```python
from build123d import *

# Parameters (mm, degrees)
BOSS_EXTRUDE1_DEPTH = 10
SKETCH2_R           = 3
CUT_EXTRUDE1_DEPTH  = 10
SKETCH4_R           = 11
CUT_EXTRUDE3_DEPTH  = 8
SKETCH5_R           = 3
SKETCH5_R_2         = 1.5
CUT_EXTRUDE4_DEPTH  = 8
SKETCH7_W           = 21.5
SKETCH7_H           = 2
BOSS_EXTRUDE2_DEPTH = 12
FILLET1_R           = 5
SKETCH8_R           = 3
CUT_EXTRUDE5_DEPTH  = 20
FILLET2_R           = 5


with BuildPart() as part:
    # Sketch1 → Boss-Extrude1 (new body)
    with BuildSketch(Plane(origin=(0, 0, 0), x_dir=(1, 0, 0), z_dir=(0, 1, 0))):
        Polygon((5.5, 11), (5.5, 26), (-26, 26), (-26, -16), (5.5, -16), (5.5, -11), (17.5, -11), (17.5, 11), align=None)
    extrude(amount=BOSS_EXTRUDE1_DEPTH)

    # Sketch2 → Cut-Extrude1 (cut)
    with BuildSketch(Plane(origin=(17.5, 0, 0), x_dir=(0, 0, -1), z_dir=(1, 0, 0))):
        with Locations((-6, 5)):
            Circle(SKETCH2_R)
        with Locations((6, 5)):
            Circle(SKETCH2_R)
    extrude(amount=-CUT_EXTRUDE1_DEPTH, mode=Mode.SUBTRACT)

    # Sketch4 → Cut-Extrude3 (cut)
    with BuildSketch(Plane.XZ):
        with Locations(Location((-11.695464036, 0, 0), (0, 0, 270))):
            Circle(SKETCH4_R)
    extrude(amount=-CUT_EXTRUDE3_DEPTH, mode=Mode.SUBTRACT)

    # Sketch5 → Cut-Extrude4 (cut)
    with BuildSketch(Plane(origin=(0, 8, 0), x_dir=(-1, 0, 0), z_dir=(0, -1, 0))):
        with Locations(Location((11.695464036, 0, 0), (0, 0, 90))):
            Circle(SKETCH5_R)
        with Locations(Location((11.695464036, -6.25, 0), (0, 0, 90))):
            Circle(SKETCH5_R_2)
        with Locations(Location((11.695464036, 6.25, 0), (0, 0, 90))):
            Circle(SKETCH5_R_2)
    extrude(amount=-CUT_EXTRUDE4_DEPTH, mode=Mode.SUBTRACT)

    # Sketch7 → Boss-Extrude2 (add)
    with BuildSketch(Plane(origin=(0, 0, 0), x_dir=(-1, 0, 0), z_dir=(0, -1, 0))):
        with Locations((10.25, 25)):
            Rectangle(SKETCH7_W, SKETCH7_H)
    extrude(amount=BOSS_EXTRUDE2_DEPTH)

    # Fillet1
    fillet1_edges = [part.edges().sort_by_distance(p)[0] for p in [
        (-26, 5, -26),
        (5.5, 5, -26),
        (5.5, 5, 16),
        (-26, 5, 16),
    ]]
    fillet(fillet1_edges, radius=FILLET1_R - 0.0001)  # a hair under: the kernel refuses the full size

    # Sketch8 → Cut-Extrude5 (cut)
    with BuildSketch(Plane.XY.offset(-24)):
        with Locations((-16, -5)):
            Circle(SKETCH8_R)
        with Locations((-4.5, -5)):
            Circle(SKETCH8_R)
    extrude(amount=-CUT_EXTRUDE5_DEPTH, mode=Mode.SUBTRACT)

    # Fillet2
    fillet2_edges = [part.edges().sort_by_distance(p)[0] for p in [
        (0.5, -12, -25),
        (-21, -12, -25),
    ]]
    fillet(fillet2_edges, radius=FILLET2_R)


solid = part.part
```
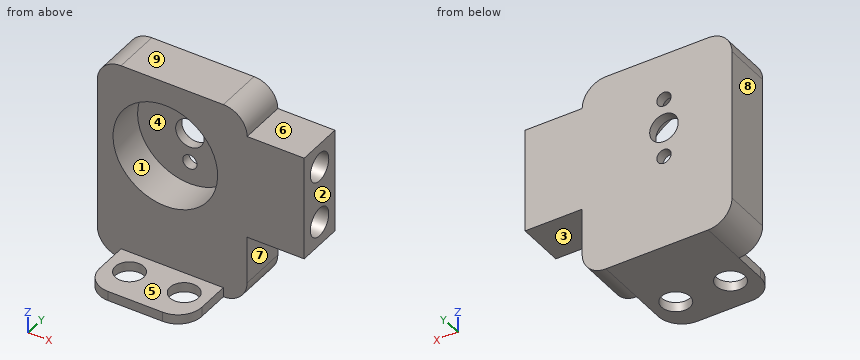
Design review of the part built by this model. Coordinates are the model's own, in mm. Face numbers are marked on the shaded views. A direction names the side the tool comes from. Give positions to 0.01 mm unless a question says otherwise; leave off trailing zeros. Order: outer loops, then holes, each group sorted by start corner. A loop starts at its lowest first (then second) coordinate and runs counter-clockwise, first axis right, second up. Notation, with made-up numbers: (-13, 52) - (24, 52) arc R17 cw to (24, 74) - close; hole circle Ø1 at (43, -15). An arc over 180 degrees is marked (long way). Use a Markdown table: item, result. Add a question column.
(1) Machinability: for the marked faces 5, 6, 7, 8 and 9, which of the approach directions +Z, -Z, +X, -X, +Y, -Y give a long, thin tool a straight path to every point of the face, cutting with its end or side? Answer none if there is none.
(2) Clearance check with flat-ended pins moving along their axes: P1, Ø1, axis at x = -6.5, y = -2, coming from the +Z side; P2, Ø13, axis at x = -11.7, z = 0, coming from the -Y side; P3, Ø12, axis at x = 1, z = 10.5, coming from the -Y side. State where each tip first meets the part, or that it passes through.
(3) Add section D-D on z = 6. Give the boundary of the cut face in (x, y) (3 decimals), then the cut area to 3 significant figures.
(4) Add section A-A on y = -5. Give the boundary of the cut face in (x, z).
(5) Add section B-B on z = 0. Give the boundary of the cut face in (x, y).
(6) Wall thickness on probe 1 along Y at (x, z) = (10, -6); probe 2 along X at (y, z) = (9.5, 0); probe 3 along X at (y, z) = (4.75, 0): over which ranges is each line inside the solid? List them lowest first. Write a range as [from, to].
(7) Mouldability with a two-part tool opening along Z and no side actions: class the marked faces 1, 2, 3 and 4 as +Z half, -Z half, draft (parallel to the pull), parting line (faces both ways), or undercut.
Report:
| question | item | result |
|---|---|---|
| 1 | face 5 | +Z, +X, -X, -Y |
| 1 | face 6 | +Z, +X, +Y, -Y |
| 1 | face 7 | -Z, +X, +Y, -Y |
| 1 | face 8 | +Z, -Z, -X, +Y, -Y |
| 1 | face 9 | +Z, +X, -X, +Y, -Y |
| 2 | P1 | stops at z = -24 |
| 2 | P2 | stops at y = 8 |
| 2 | P3 | stops at y = 0 |
| 3 | outline | (-26, 0) - (-20.915, 0) - (-20.915, 8) - (-13.174, 8) - (-13.174, 10) - (-26, 10) - close; (-10.216, 8) - (-2.476, 8) - (-2.476, 0) - (17.5, 0) - (17.5, 2) - (7.5, 2) - (7.5, 8) - (17.5, 8) - (17.5, 10) - (-10.216, 10) - close |
| 3 | area | 222 mm² |
| 4 | outline | (-21, -26) - (-19, -26) - (-19, -24) - (-21, -24) - close; (-13, -26) - (-7.5, -26) - (-7.5, -24) - (-13, -24) - close; (-1.5, -26) - (0.5, -26) - (0.5, -24) - (-1.5, -24) - close |
| 5 | outline | (-26, 0) - (-22.7, 0) - (-22.7, 8) - (-14.7, 8) - (-14.7, 10) - (-26, 10) - close; (-8.7, 8) - (-0.7, 8) - (-0.7, 0) - (17.5, 0) - (17.5, 10) - (-8.7, 10) - close |
| 6 | probe 1 | y = [0, 2], [8, 10] |
| 6 | probe 2 | x = [-26, -14.7], [-8.7, 17.5] |
| 6 | probe 3 | x = [-26, -22.7], [-0.7, 17.5] |
| 7 | face 1 | undercut |
| 7 | face 2 | draft |
| 7 | face 3 | -Z half |
| 7 | face 4 | undercut |
